Build history of the part. All positions in model axes, mm. Face numbers are marked on the shaded views. Round coordinates to 2 decimals unless told otherwise and drop trailing zeros. Order: outer loops, then holes, each group sorted by start corner. A loop starts at its lowest first (then second) coordinate and runs counter-clockwise, first axis right, second up. Notation, with made-up numbers: (-6.5, 48.25) - (21.5, 48.25) arc R25 cw to (21.5, 87.25) - close; hole circle Ø1 at (21.5, -9.5). An arc over 180 degrees is marked (long way). One line per question, with ' | ' between items. Start each with the question number.
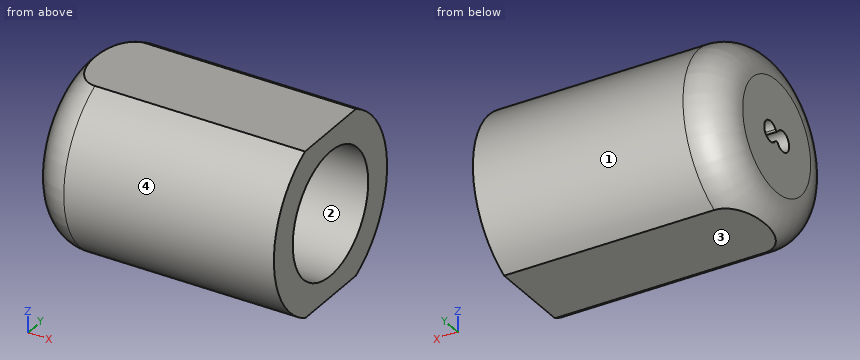
from build123d import *

# Parameters (mm, degrees)
FILLET1_R          = 3
SKETCH2_W          = 17.193533638
SKETCH2_H          = 22.71470374
SKETCH2_W_2        = 13.4
SKETCH2_H_2        = 17.458798434
CUT_EXTRUDE1_DEPTH = 23.638462845
CUT_EXTRUDE3_DEPTH = 21.618923503


with BuildPart() as part:
    # Sketch1 → Revolve1 (revolve)
    with BuildSketch(Plane.XY, mode=Mode.PRIVATE) as revolve1_sk:
        Polygon((18, 7.5), (18, 5), (0, 5), (0, 0), (-2, 0), (-2, 7.5), align=None)
    revolve(revolve1_sk.sketch.rotate(Axis((-2, 0, 0), (1, 0, 0)), 90), axis=Axis((-2, 0, 0), (1, 0, 0)))

    # Fillet1
    fillet1_edges = [part.edges().sort_by_distance(p)[0] for p in [
        (-2, 0, -7.5),
    ]]
    fillet(fillet1_edges, radius=FILLET1_R)

    # Sketch2 → Cut-Extrude1 (cut, through all)
    with BuildSketch(Plane(origin=(18, 0, 0), x_dir=(0, 0, -1), z_dir=(1, 0, 0))):
        Rectangle(SKETCH2_W, SKETCH2_H)
        Rectangle(SKETCH2_W_2, SKETCH2_H_2, mode=Mode.SUBTRACT)
    extrude(amount=-CUT_EXTRUDE1_DEPTH, mode=Mode.SUBTRACT)

    # Sketch3 → Cut-Extrude3 (cut, through all)
    with BuildSketch(Plane(origin=(0, 0, 0), x_dir=(0, 0, -1), z_dir=(1, 0, 0))):
        with BuildLine():
            ThreePointArc((0.489588204, 0.16097561), (0, 1.65), (-0.489588204, 0.16097561))
            ThreePointArc((-0.489588204, 0.16097561), (-0.408276253, 0), (-0.489588204, -0.16097561))
            ThreePointArc((-0.489588204, -0.16097561), (0, -1.65), (0.489588204, -0.16097561))
            ThreePointArc((0.489588204, -0.16097561), (0.408276253, 0), (0.489588204, 0.16097561))
        make_face()
    extrude(amount=-CUT_EXTRUDE3_DEPTH, mode=Mode.SUBTRACT)


solid = part.part
Item 1: Pin check, flat tips, straight feed: pin 1 (1.5 mm diameter, centred on x = 10.5, z = -2, fed in from +Y); pin 2 (1.5 mm diameter, centred on x = 4, z = 4, fed in from +Y); pin 3 (2 mm diameter, centred on x = 4, z = 4.5, fed in from -Y). Stop position of each tip, or through.
Item 2: Slice it at B-B (x = 2). Write the cut outline in (y, z).
Item 3: Slice it at A-A (z = 0). Write the cut outline in (x, y).
Item 4: Wall check: line 1 along Y through (x, z) = (12.25, 0); line 2 along Z through (x, y) = (3.5, 6); line 3 along Z through (x, y) = (13.5, 2.75). Give the ranges that are in metal, low to high. Write a range as [from, to].
Item 5: Pull direction Y, two halves, no side cores. Call the marked faces 1, 2, 3 and 4: released by +Y, released by -Y, zero draft, split by the parting line, or undercut.
A:
1) pin 1: y = 7.4 | pin 2: y = 6.76 | pin 3: y = -6.63
2) outline: (-3.37, -6.7) - (3.37, -6.7) arc R7.5 ccw to (3.37, 6.7) - (-3.37, 6.7) arc R7.5 ccw to start; hole circle Ø10 at (0, 0)
3) outline: (-2, -4.5) arc R3 ccw to (1, -7.5) - (18, -7.5) - (18, -5) - (0, -5) - (0, -1.65) - (-2, -1.65) - close; (-2, 1.65) - (0, 1.65) - (0, 5) - (18, 5) - (18, 7.5) - (1, 7.5) arc R3 ccw to (-2, 4.5) - close
4) line 1: [-7.5, -5], [5, 7.5] | line 2: [-4.5, 4.5] | line 3: [-6.7, -4.18], [4.18, 6.7]
5) face 1: released by +Y | face 2: undercut | face 3: zero draft | face 4: released by -Y
